```python
from build123d import *

# Parameters (mm, degrees)
F2_R     = 8.9916
F3_DEPTH = 3.556
F5_DEPTH = 1.778


with BuildPart() as f1:
    # F0 (on Front) → F1 (revolve)
    with BuildSketch(Plane.XZ):
        with BuildLine():
            Line((-10.16, 0), (0, 0))
            Line((0, 0), (0, 31.242))
            Line((0, 31.242), (-9.7536, 31.242))
            Line((-9.7536, 31.242), (-9.7536, 26.162))
            ThreePointArc((-9.7536, 26.162), (-6.161498, 24.674102), (-4.6736, 21.082))
            Line((-4.6736, 21.082), (-4.445, 5.842))
            ThreePointArc((-4.445, 5.842), (-4.519395, 5.662395), (-4.699, 5.588))
            ThreePointArc((-4.699, 5.588), (-4.878605, 5.513605), (-4.953, 5.334))
            Line((-4.953, 5.334), (-5.08, 5.334))
            Line((-5.08, 5.334), (-5.08, 5.08))
            ThreePointArc((-5.08, 5.08), (-8.672102, 3.592102), (-10.16, 0))
        make_face()
    revolve(axis=Axis((0, 0, 15.621), (0, 0, -1)))

    # F2 (on face) → F3 (cut)
    with BuildSketch(Plane.XY.offset(31.242)):
        Circle(F2_R)
    extrude(amount=-F3_DEPTH, mode=Mode.SUBTRACT)

    # F4 (on face) → F5 (cut)
    with BuildSketch(Plane.XY.offset(31.242)):
        Polygon((-0.508, -0.508), (-0.508, 0), (-0.508, 0.508), (-8.064261, 0.508), (-8.064261, -0.508), align=None)
        Polygon((-0.508, 6.998243), (-0.508, 0.508), (0, 0.508), (0.508, 0.508), (0.508, 6.998243), align=None)
        Polygon((0, -0.508), (-0.508, -0.508), (-0.508, -7.178504), (0.508, -7.178504), (0.508, -0.508), align=None)
        Polygon((0.508, 0.508), (0.508, 0), (0.508, -0.508), (7.389117, -0.508), (7.389117, 0.508), align=None)
    extrude(amount=-F5_DEPTH, mode=Mode.SUBTRACT)


solid = f1.part
```
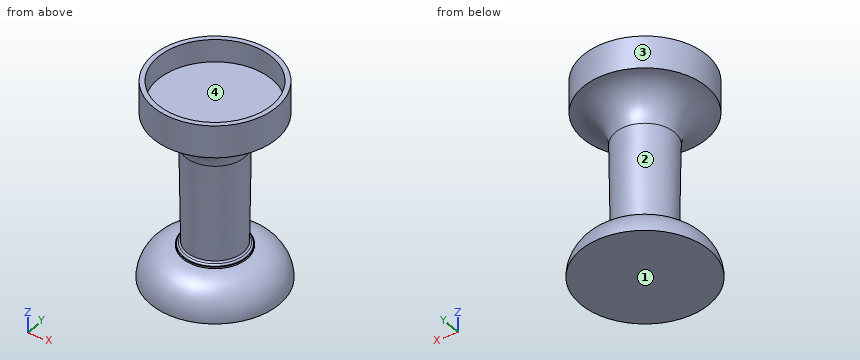
Model file for the job. Use its own axes, mm. Face numbers are marked on the shaded views. Coordinates: 2 decimals unless noted, no trailing zeros. Write each loop counter-clockwise with the first axis right and the second up, starting at its lowest first coordinate (ties: lowest second). Pieces come first, ordered by that corner, then holes. Notation, with made-up numbers: (-21.5, 71) - (-0.5, 71) arc R29 cw to (-0.5, 93) - close; hole circle Ø11 at (37.25, 75.25). An arc over 180 degrees is marked (long way). One line per item, written item: value. Start each with the question number.
1. Probe line 1 (Y direction, x = 0, z = 29.9); line 2 (Z direction, x = -4.25, y = -5.5); line 3 (Z direction, x = -1.5, y = 3.5). List the from-to ranges inside material, lowest first. Write a range as from..to.
2. Slice it at B-B (z = 15). Write the cut outline in (x, y).
3. Slice it at C-C (z = 19.5). Write the cut outline in (x, y).
4. Slice it at A-A (z = 29). Write the cut outline in (x, y), plus the area to 3 significant figures.
5. Flat gauge pins, fed straight in: pin 1 (3 mm diameter, centred on x = -3, z = 4.5, fed in from +Y); pin 2 (1.5 mm diameter, centred on x = -4, y = -8, fed in from -Z); pin 3 (3 mm diameter, centred on y = -2.5, z = 17.5, fed in from +X); pin 4 (2 mm diameter, centred on x = 3.5, z = 16.5, fed in from -Y). Where does each tip first touch, or does it go through?
6. Mould opens along Z. For the marked faces 1, 2, 3 and 4 say: released by +Z, released by -Z, zero draft, split by the parting line, or undercut.
Answers below:
1. line 1: y = -9.75..-8.99, 8.99..9.75
1. line 2: z = 0..4.72, 25.32..27.69
1. line 3: z = 0..27.69
2. outline: circle Ø9.16 at (0, 0)
3. outline: circle Ø9.3 at (0, 0)
4. outline: circle Ø19.51 at (0, 0); hole circle Ø17.98 at (0, 0)
4. area: 44.9 mm^2
5. pin 1: stops at y = 8.77
5. pin 2: stops at z = 0
5. pin 3: stops at x = 4.51
5. pin 4: stops at y = -3.87
6. face 1: released by -Z
6. face 2: undercut
6. face 3: zero draft
6. face 4: released by +Z
